Could you check a few things on this drawing? It's one solid part, dimensions in mm from its lowest x, y, z. A direction names the side the tool comes from. Give positions to 0.01 mm unless a question says otherwise; leave off trailing zeros. Loops run counter-clockwise (first coordinate to the right, second up) from the corner with the lowest first, then second, coordinate; pieces in that order, holes last.
1. Imagine slicing it at C-C (z = 37.5). List the corners of the cut face in (x, y) for me, plus the area to 3 significant figures.
2. For P1, Ø0.9, axis at x = 57, y = 4, coming from the +Z side; P2, Ø1.8, axis at y = 3, z = 38, coming from the -X side; P3, Ø3, axis at y = 4, z = 39, coming from the +X side, each with a flat end and sliding along its axis, tell me the tip position at first contact or that it passes through.
3. Imagine slicing it at B-B (y = 0.9). List the corners of the cut face in (x, z) for me, plus the area to 4 significant figures.
4. Imagine slicing it at A-A (z = 7). List the corners of the cut face in (x, y) for me, plus the area to 3 significant figures.
5. For the marked faces 1, 2 and 3, which set-ups out of +Z, -Z, +X, -X, +Y, -Y let a thin tool reach every point of the face, with its end or its side?
6. I need wall thicknesses on line 1 along X through (y, z) = (2.15, 37.5); line 2 along Y through (x, z) = (5.75, 3.75); line 3 along X through (y, z) = (3.8, 10.5). Which ranges of each line are inside material? Lowest first, please.
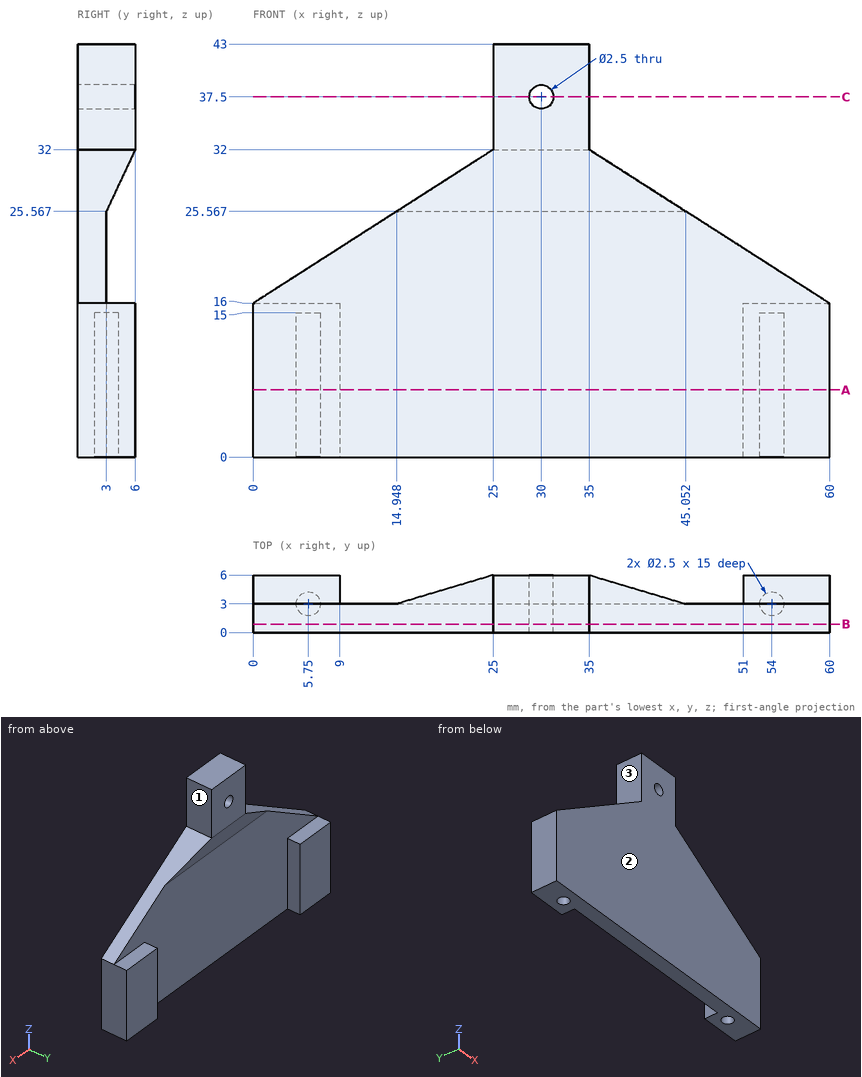
Derived:
1. outline: (25, 0) - (28.75, 0) - (28.75, 6) - (25, 6) - close; (31.25, 0) - (35, 0) - (35, 6) - (31.25, 6) - close
1. area: 45.0 mm2
2. P1: stops at z = 16
2. P2: stops at x = 25
2. P3: stops at x = 35
3. outline: (0, 0) - (60, 0) - (60, 16) - (35, 32) - (35, 43) - (25, 43) - (25, 32) - (0, 16) - close; hole circle Ø2.5 at (30, 37.5)
3. area: 1,625 mm2
4. outline: (0, 0) - (60, 0) - (60, 6) - (51, 6) - (51, 3) - (9, 3) - (9, 6) - (0, 6) - close; hole circle Ø2.5 at (5.75, 3); hole circle Ø2.5 at (54, 3)
4. area: 224 mm2
5. face 1: +Z, +X, +Y, -Y
5. face 2: +Z, -Z, +X, -X, -Y
5. face 3: +Z, -X, +Y, -Y
6. line 1: x = 25 to 28.75, 31.25 to 35
6. line 2: y = 0 to 1.75, 4.25 to 6
6. line 3: x = 0 to 4.79, 6.71 to 9, 51 to 53.04, 54.96 to 60
